Autodesk Inventor part; units mm, degrees
ref_plane "YZ Plane" through (0, 0, 0) normal (1, 0, 0) x (0, 1, 0)
ref_plane "XZ Plane" through (0, 0, 0) normal (0, 1, 0) x (-1, 0, 0)
ref_plane "XY Plane" through (0, 0, 0) normal (0, 0, 1) x (1, 0, 0)
sketch "스케치1" plane through (0, 0, 0) normal (0, 1, 0) x (-1, 0, 0)
  line L0 (100, -100) -> (-100, -100)
  line L1 (-100, -100) -> (-100, 100)
  line L2 (-100, 100) -> (100, 100)
  line L3 (100, 100) -> (100, -100)
  line L4 (100, -100) -> (-100, 100) construction
  line L5 (-100, -100) -> (100, 100) construction
  point P0 (0, 0)
  dimension "d0" = 200
  dimension "d1" = 200
extrude "돌출1" add sketch "스케치1" along normal blind 200
sketch "스케치2" plane through (0, 200, 0) normal (0, 1, 0) x (1, 0, 0)
  line L0 (-95, 95) -> (95, 95)
  line L1 (95, 95) -> (95, -95)
  line L2 (95, -95) -> (-95, -95)
  line L3 (-95, -95) -> (-95, 95)
  line L4 (-95, 95) -> (95, -95) construction
  line L5 (95, 95) -> (-95, -95) construction
  point P0 (0, 0)
  dimension "d4" = 190
  dimension "d5" = 190
extrude "돌출2" cut sketch "스케치2" against normal blind 195
properties part number "safe"
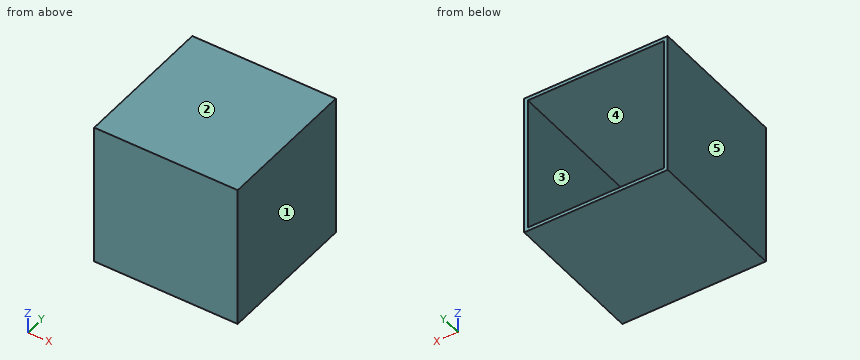
Check sheet for the modelled part. Datum: model origin and axes. Units: mm. Face numbers are marked on the shaded views. A direction names the side the tool comes from. Give positions to 0.01 mm unless a question says otherwise; leave off trailing zeros. Loops run counter-clockwise (first coordinate to the right, second up) from the corner with the lowest first, then second, coordinate; pieces in that order, holes last. Notation, with made-up numbers: M 81,46 L 117,46 A22 cw 117,80 Z; hole C 86.25,68 d9. An arc over 180 degrees is marked long. Use a Markdown table: item, result. Add a question column.
Q1. Sectioned sample at A-A, the plane y = 23. Record the cut outline in (x, z), then the cut area to 3 significant figures.
Q2. Mould release check, pull along X, two halves, no side actions. Record for the marked faces 1, 2 and 3: pulls with the +X half, pulls with the -X half, needs draft (parallel to the pull), parting line crosses it, or undercut.
Q3. Scan lines: line 1 along X through (y, z) = (92.5, -58); line 2 along Y through (x, z) = (47.5, 23). Record each from-to range of solid material in increasing order. Write a range as [from, to].
Q4. Go/stop test with a flat-tipped pin: pin 1 (5 mm diameter, centred on x = -65, z = -22.5, fed in from +Y). Record where the tip stops, or that it passes through.
Q5. Sectioned sample at C-C, the plane z = -87. Record the cut outline in (x, y).
Q6. Sectioned sample at B-B, the plane x = -79.5. Record the cut outline in (y, z), then the cut area to 3 significant figures.
Q7. Tool access check on the marked faces 4 and 5. Record the directions out of +Z, -Z, +X, -X, +Y, -Y that give a thin tool (end or side, any length) a straight path to the whole face; none if there is none.
Verdict:
| question | item | result |
|---|---|---|
| 1 | outline | M -100,-100 L 100,-100 L 100,100 L -100,100 Z; hole M -95,-95 L 95,-95 L 95,95 L -95,95 Z |
| 1 | area | 3,900 mm^2 |
| 2 | face 1 | pulls with the +X half |
| 2 | face 2 | needs draft |
| 2 | face 3 | undercut |
| 3 | line 1 | [-100, -95], [95, 100] |
| 3 | line 2 | [0, 5] |
| 4 | pin 1 | y = 5 |
| 5 | outline | M -100,0 L 100,0 L 100,200 L 95,200 L 95,5 L -95,5 L -95,200 L -100,200 Z |
| 6 | outline | M 0,-100 L 200,-100 L 200,-95 L 5,-95 L 5,95 L 200,95 L 200,100 L 0,100 Z |
| 6 | area | 2,950 mm^2 |
| 7 | face 4 | +Y |
| 7 | face 5 | +Z, -Z, -X, +Y, -Y |
